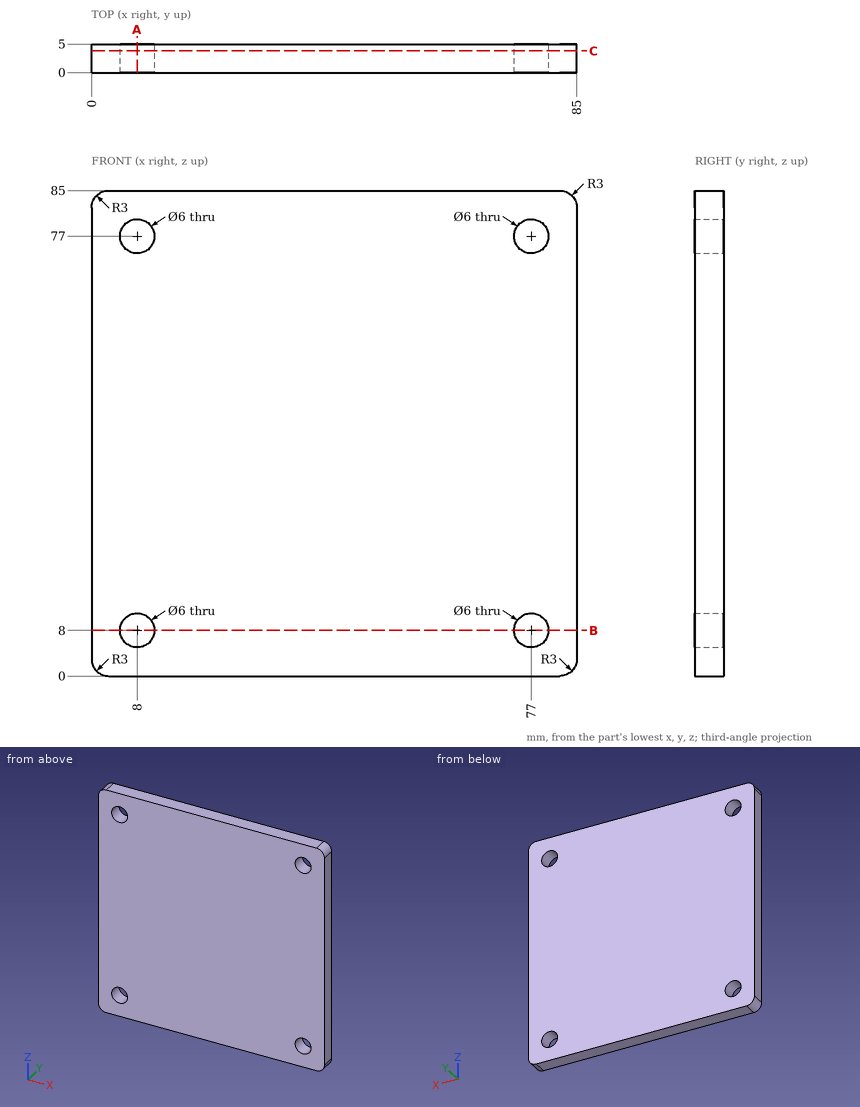
Verification items for this drawing (mm, ordinates from the low corner). Coordinates: 2 decimals unless noted, no trailing zeros. Loops run counter-clockwise (first coordinate to the right, second up) from the corner with the lowest first, then second, coordinate; pieces in that order, holes last. Notation, with made-up numbers: (44, 6) - (97, 6) arc R19 cw to (97, 10) - close; hole circle Ø8 at (30.25, -20). An arc over 180 degrees is marked (long way). One line per item, written item: value. Start each with the question number.
(1) Material ranges on line 1 (Z direction, x = 77, y = 3.1); line 2 (Z direction, x = 76, y = 2.65), recorded low to high. Write a range as [from, to].
(2) Cross-section at A-A on x = 8. Enter the section's corners in (y, z), plus the area to 3 significant figures.
(3) Cross-section at C-C on y = 3.8. Enter the section's corners in (x, z), plus the area to 3 significant figures.
(4) Depth check by flat-ended pin: P1, Ø5.5, axis at x = 8, z = 77, coming from the +Y side. Enter the tip coordinate at first touch or a pass-through.
(5) Cross-section at B-B on z = 8. Enter the section's corners in (x, y), plus the area to 3 significant figures.
Results below:
1. line 1: z = [0, 5], [11, 74], [80, 85]
1. line 2: z = [0, 5.17], [10.83, 74.17], [79.83, 85]
2. outline: (0, 0) - (5, 0) - (5, 5) - (0, 5) - close; (0, 11) - (5, 11) - (5, 74) - (0, 74) - close; (0, 80) - (5, 80) - (5, 85) - (0, 85) - close
2. area: 365 mm2
3. outline: (0, 3) arc R3 ccw to (3, 0) - (82, 0) arc R3 ccw to (85, 3) - (85, 82) arc R3 ccw to (82, 85) - (3, 85) arc R3 ccw to (0, 82) - close; hole circle Ø6 at (8, 8); hole circle Ø6 at (8, 77); hole circle Ø6 at (77, 8); hole circle Ø6 at (77, 77)
3. area: 7,100 mm2
4. P1: passes through
5. outline: (0, 0) - (5, 0) - (5, 5) - (0, 5) - close; (11, 0) - (74, 0) - (74, 5) - (11, 5) - close; (80, 0) - (85, 0) - (85, 5) - (80, 5) - close
5. area: 365 mm2
